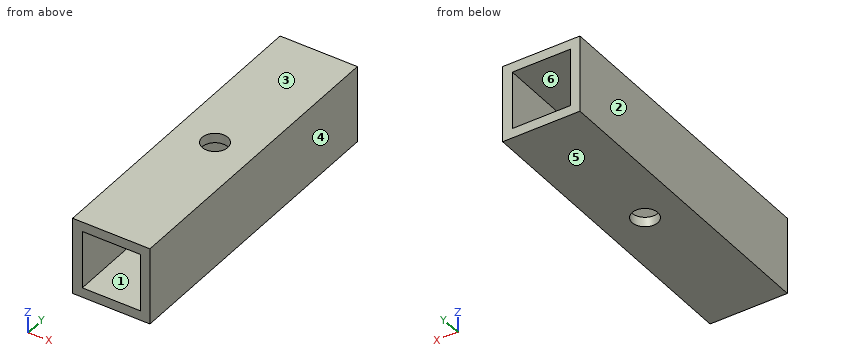
from build123d import *

# Parameters (mm, degrees)
SKETCH1_W                  = 38.1
SKETCH1_H                  = 38.1
SKETCH1_W_2                = 28.575
SKETCH1_H_2                = 28.575
BOSS_EXTRUDE1_DEPTH        = 152.4
F_1_2_0_5_DIAMETER_HOLE1_D = 12.7


with BuildPart() as part:
    # Sketch1 → Boss-Extrude1 (new body)
    with BuildSketch(Plane(origin=(0, 0, 0), x_dir=(1, 0, 0), z_dir=(0, 1, 0))):
        with Locations((19.05, 19.05)):
            Rectangle(SKETCH1_W, SKETCH1_H)
        with Locations((19.05, 19.05)):
            Rectangle(SKETCH1_W_2, SKETCH1_H_2, mode=Mode.SUBTRACT)
    extrude(amount=BOSS_EXTRUDE1_DEPTH)

    # 1/2 (0.5) Diameter Hole1 (through all)
    with Locations(Plane.XY):
        with Locations((19.05, 76.2)):
            Hole(F_1_2_0_5_DIAMETER_HOLE1_D / 2)


solid = part.part
Model file for the job. Use its own axes, mm. Face numbers are marked on the shaded views. A direction names the side the tool comes from. Give positions to 0.01 mm unless a question says otherwise; leave off trailing zeros. Order: outer loops, then holes, each group sorted by start corner. A loop starts at its lowest first (then second) coordinate and runs counter-clockwise, first axis right, second up. Notation, with made-up numbers: (-10.75, 75.5) - (8.25, 75.5) arc R17 ccw to (8.25, 85.5) - close; hole circle Ø10 at (83, 0). An arc over 180 degrees is marked (long way). Write item = value, one per line. Start each with the question number.
1. Probe line 1 along Y through (x, z) = (19, -36); line 2 along Z through (x, y) = (31.5, 104.5); line 3 along X through (y, z) = (105, -16.5). List the from-to ranges inside material, lowest first.
2. Cut at A-A, the plane x = 19.05. List the corners of the cut face in (y, z).
3. Cut at C-C, the plane x = 31.5. List the corners of the cut face in (y, z).
4. Cut at D-D, the plane y = 76.2. List the corners of the cut face in (x, z), and give its area (3 significant figures).
5. Cut at B-B, the plane z = -13.5. List the corners of the cut face in (x, y), and give its area (3 significant figures).
6. Two-plate mould, pull along Z, no slides. Class the marked faces 3, 4, 5 and 6: pulls with the +Z half, pulls with the -Z half, needs draft (parallel to the pull), parting line crosses it, or undercut.
7. Which spindle directions (+Z, -Z, +X, -X, +Y, -Y) get a long thin tool onto all of the face, cutting with end or side? Do the marked faces 1 and 2. Say none if no direction does.
Taken from the geometry:
q1.line_1 = 0 to 69.85, 82.55 to 152.4
q1.line_2 = -38.1 to -33.34, -4.76 to 0
q1.line_3 = 0 to 4.76, 33.34 to 38.1
q2.outline = (0, -38.1) - (69.85, -38.1) - (69.85, -33.34) - (0, -33.34) - close; (0, -4.76) - (69.85, -4.76) - (69.85, 0) - (0, 0) - close; (82.55, -38.1) - (152.4, -38.1) - (152.4, -33.34) - (82.55, -33.34) - close; (82.55, -4.76) - (152.4, -4.76) - (152.4, 0) - (82.55, 0) - close
q3.outline = (0, -38.1) - (152.4, -38.1) - (152.4, -33.34) - (0, -33.34) - close; (0, -4.76) - (152.4, -4.76) - (152.4, 0) - (0, 0) - close
q4.outline = (0, -38.1) - (12.7, -38.1) - (12.7, -33.34) - (4.76, -33.34) - (4.76, -4.76) - (12.7, -4.76) - (12.7, 0) - (0, 0) - close; (25.4, -38.1) - (38.1, -38.1) - (38.1, 0) - (25.4, 0) - (25.4, -4.76) - (33.34, -4.76) - (33.34, -33.34) - (25.4, -33.34) - close
q4.area = 514 mm²
q5.outline = (0, 0) - (4.76, 0) - (4.76, 152.4) - (0, 152.4) - close; (33.34, 0) - (38.1, 0) - (38.1, 152.4) - (33.34, 152.4) - close
q5.area = 1,450 mm²
q6.face_3 = pulls with the +Z half
q6.face_4 = needs draft
q6.face_5 = pulls with the -Z half
q6.face_6 = undercut
q7.face_1 = +Y, -Y
q7.face_2 = +Z, -Z, -X, +Y, -Y
